from build123d import *

# Parameters (mm, degrees)
F0_R     = 11.2
F1_DEPTH = 7
F3_DEPTH = 1


with BuildPart() as f1:
    # F0 (on Top) → F1 (new body)
    with BuildSketch(Plane.XY):
        Polygon((25.6720134951, 14.5481945947), (-25.6720134951, 14.5481945947), (-37.758209943, 0), (0, -34.8202470113), (37.758209943, 0), align=None)
        with Locations((0, -3.7951807026)):
            Circle(F0_R, mode=Mode.SUBTRACT)
    extrude(amount=F1_DEPTH)

    # F2 (on face) → F3 (join)
    with BuildSketch(Plane.XY.offset(7)):
        with BuildLine():
            add(Edge.make_bspline(
                [(14.7238187039, -15.7416694783), (14.7238187039, -20.8010980146), (11.6681145092, -24.0600274463)],
                knots=[0, 0, 0, 0.8391754789, 0.8391754789, 0.8391754789], degree=2))
            add(Edge.make_bspline(
                [(12.410573631, -8.3928551309), (14.7238187039, -11.3878987516), (14.7238187039, -15.7416694783)],
                knots=[0, 0, 0, 1, 1, 1], degree=2))
            add(Edge.make_bspline(
                [(10.8114000869, -6.7198393426), (11.7643435247, -7.5561572037), (12.410573631, -8.3928551309)],
                knots=[0.7206391515, 0.7206391515, 0.7206391515, 1, 1, 1], degree=2))
            ThreePointArc((10.8114000869, -6.7198393426), (8.586875435, -10.9858392444), (4.7778268514, -13.9249571353))
            add(Edge.make_bspline(
                [(5.4708384123, -16.1994485033), (5.4708384123, -14.9282205842), (4.7778268514, -13.9249571353)],
                knots=[0, 0, 0, 0.9740036675, 0.9740036675, 0.9740036675], degree=2))
            add(Edge.make_bspline(
                [(3.8101719494, -19.730190983), (5.4708384123, -18.5467835036), (5.4708384123, -16.1994485033)],
                knots=[0, 0, 0, 1, 1, 1], degree=2))
            add(Edge.make_bspline(
                [(-0.9478079163, -20.9135984624), (2.1495054866, -20.9135984624), (3.8101719494, -19.730190983)],
                knots=[0, 0, 0, 1, 1, 1], degree=2))
            add(Edge.make_bspline(
                [(-6.660305749, -20.095440205), (-3.538642398, -20.9135984624), (-0.9478079163, -20.9135984624)],
                knots=[0, 0, 0, 1, 1, 1], degree=2))
            add(Edge.make_bspline(
                [(-14.2818395155, -17.261106242), (-9.7819691, -19.2772819476), (-6.660305749, -20.095440205)],
                knots=[0, 0, 0, 1, 1, 1], degree=2))
            Line((-14.2818395155, -17.261106242), (-14.2818395155, -21.6496761485))
            Line((-14.2818395155, -21.6496761485), (-7.0797239554, -28.2913957424))
            add(Edge.make_bspline(
                [(-1.6783063604, -28.7153218451), (-4.5095721098, -28.7153218451), (-7.0797239554, -28.2913957424)],
                knots=[0, 0, 0, 0.3971106389, 0.3971106389, 0.3971106389], degree=2))
            add(Edge.make_bspline(
                [(10.3846579461, -25.2430192409), (6.0454971883, -28.7153218451), (-1.6783063604, -28.7153218451)],
                knots=[0, 0, 0, 1, 1, 1], degree=2))
            add(Edge.make_bspline(
                [(10.389586169, -25.239073611), (10.3871227576, -25.2410468384), (10.3846579461, -25.2430192409)],
                knots=[0.9994319612, 0.9994319612, 0.9994319612, 1, 1, 1], degree=2))
            Line((10.389586169, -25.239073611), (11.6681145092, -24.0600274463))
        make_face()
        with BuildLine():
            add(Edge.make_bspline(
                [(12.9648102038, 14.5481945947), (13.729785447, 14.2447942788), (14.5095391603, 13.9068273719)],
                knots=[0.7732095753, 0.7732095753, 0.7732095753, 1, 1, 1], degree=2))
            Line((12.9648102038, 14.5481945947), (-8.5649794853, 14.5481945947))
            add(Edge.make_bspline(
                [(-9.7624891415, 13.6584579009), (-9.1945173533, 14.1372954304), (-8.5649794853, 14.5481945947)],
                knots=[0, 0, 0, 0.1418818722, 0.1418818722, 0.1418818722], degree=2))
            add(Edge.make_bspline(
                [(-13.765620615, 4.3713876819), (-13.765620615, 10.2835550893), (-9.7624891415, 13.6584579009)],
                knots=[0, 0, 0, 1, 1, 1], degree=2))
            add(Edge.make_bspline(
                [(-12.5481232082, -1.102480659), (-13.765620615, 1.2448543413), (-13.765620615, 4.3713876819)],
                knots=[0, 0, 0, 1, 1, 1], degree=2))
            add(Edge.make_bspline(
                [(-11.1855575293, -3.2265835185), (-11.962161159, -2.23221549), (-12.5481232082, -1.102480659)],
                knots=[0.5187159775, 0.5187159775, 0.5187159775, 1, 1, 1], degree=2))
            ThreePointArc((-11.1855575293, -3.2265835185), (-9.1028902875, 2.7299544235), (-4.1307340981, 6.6152484822))
            add(Edge.make_bspline(
                [(-3.1100833108, 7.936220089), (-3.7746308536, 7.3575664463), (-4.1307340981, 6.6152484822)],
                knots=[0, 0, 0, 0.4641418083, 0.4641418083, 0.4641418083], degree=2))
            add(Edge.make_bspline(
                [(1.0001879346, 9.1829374336), (-1.6783063604, 9.1829374336), (-3.1100833108, 7.936220089)],
                knots=[0, 0, 0, 1, 1, 1], degree=2))
            add(Edge.make_bspline(
                [(5.5779781841, 8.6034086679), (3.2501231423, 9.1829374336), (1.0001879346, 9.1829374336)],
                knots=[0, 0, 0, 1, 1, 1], degree=2))
            add(Edge.make_bspline(
                [(11.470665633, 6.5628830141), (7.9058332259, 8.0238799023), (5.5779781841, 8.6034086679)],
                knots=[0, 0, 0, 1, 1, 1], degree=2))
            Line((11.470665633, 6.5628830141), (14.5095391603, 13.9068273719))
        make_face()
    extrude(amount=F3_DEPTH)


solid = f1.part
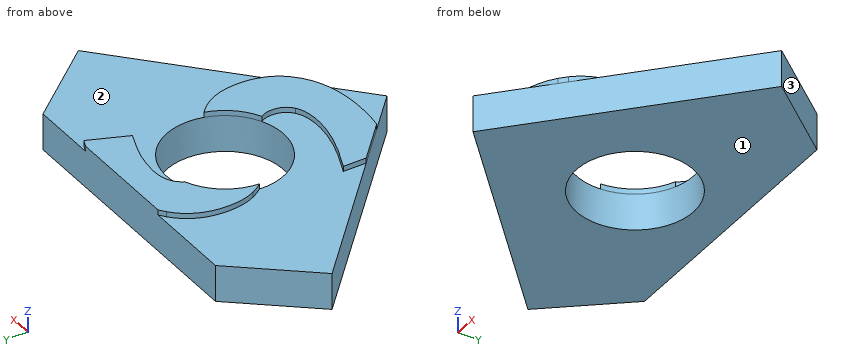
For this review, take the finished solid that the model builds, in its own axes (mm). Face numbers are marked on the shaded views. Round coordinates to 2 decimals unless told otherwise and drop trailing zeros. Write each loop counter-clockwise with the first axis right and the second up, starting at its lowest first coordinate (ties: lowest second). Pieces come first, ordered by that corner, then holes. Notation, with made-up numbers: (29, 76) - (62, 76) arc R23 ccw to (62, 85) - close; hole circle Ø7 at (1, 56). An arc over 180 degrees is marked (long way). Use a Markdown table: item, result.
Q1. Clearance check with flat-ended pins moving along their axes: pin 1 (4 mm diameter, centred on y = -24.5, z = 4, fed in from +X); pin 2 (2 mm diameter, centred on y = -9.5, z = 2, fed in from +X); pin 3 (0.5 mm diameter, centred on y = -20.5, z = 7.5, fed in from -X). State where each tip first meets the part, or that it passes through.
Derived:
| item | result |
|---|---|
| pin 1 | stops at x = 13.36 |
| pin 2 | stops at x = 28.54 |
| pin 3 | stops at x = -14.28 |
Q2. We need section B-B (x = 22). Give the boundary of the cut face in (y, z), plus the area to 3 significant figures.
Derived:
| item | result |
|---|---|
| outline | (-14.53, 0) - (14.55, 0) - (14.55, 7) - (-14.53, 7) - close |
| area | 204 mm2 |
Q3. We need section A-A (z = 2). Give the boundary of the cut face in (x, y), plus the area to 3 significant figures.
Derived:
| item | result |
|---|---|
| outline | (-37.76, 0) - (0, -34.82) - (37.76, 0) - (25.67, 14.55) - (-25.67, 14.55) - close; hole circle Ø22.4 at (0, -3.8) |
| area | 1,840 mm2 |
Q4. The part is to be moulded in two halves that separate along Z. For the marked faces 1, 2 and 3, say which applies: pulls with the +Z half, pulls with the -Z half, needs draft (parallel to the pull), parting line crosses it, or undercut.
Derived:
| item | result |
|---|---|
| face 1 | pulls with the -Z half |
| face 2 | pulls with the +Z half |
| face 3 | needs draft |
Q5. We need section C-C (x = -32.5). Give the boundary of the cut face in (y, z).
Derived:
| item | result |
|---|---|
| outline | (-4.85, 0) - (6.33, 0) - (6.33, 7) - (-4.85, 7) - close |
Q6. Wall thickness on line 1 along Y through (x, z) = (0, 3); line 2 along X through (y, z) = (-11, 0.5) (3 decimals); line 3 along Z through (x, y) = (-3, -19.5): over which ranges is each line inside the solid? List them lowest first.
Derived:
| item | result |
|---|---|
| line 1 | y = -34.82 to -15, 7.4 to 14.55 |
| line 2 | x = -25.83 to -8.575, 8.575 to 25.83 |
| line 3 | z = 0 to 7 |
